The figure shows three views and two pictorial views of one solid part (mm, origin at its lowest corner). Answer the questions. A direction names the side the tool comes from. Round coordinates to 2 decimals unless told otherwise and drop trailing zeros. Order: outer loops, then holes, each group sorted by start corner. A loop starts at its lowest first (then second) coordinate and runs counter-clockwise, first axis right, second up. Notation, with made-up numbers: (-10, 44) - (2, 44) arc R6 ccw to (2, 49) - close; hole circle Ø9 at (86.25, 89). An arc over 180 degrees is marked (long way). Use CSV: the item, a comma, the result in double quotes.
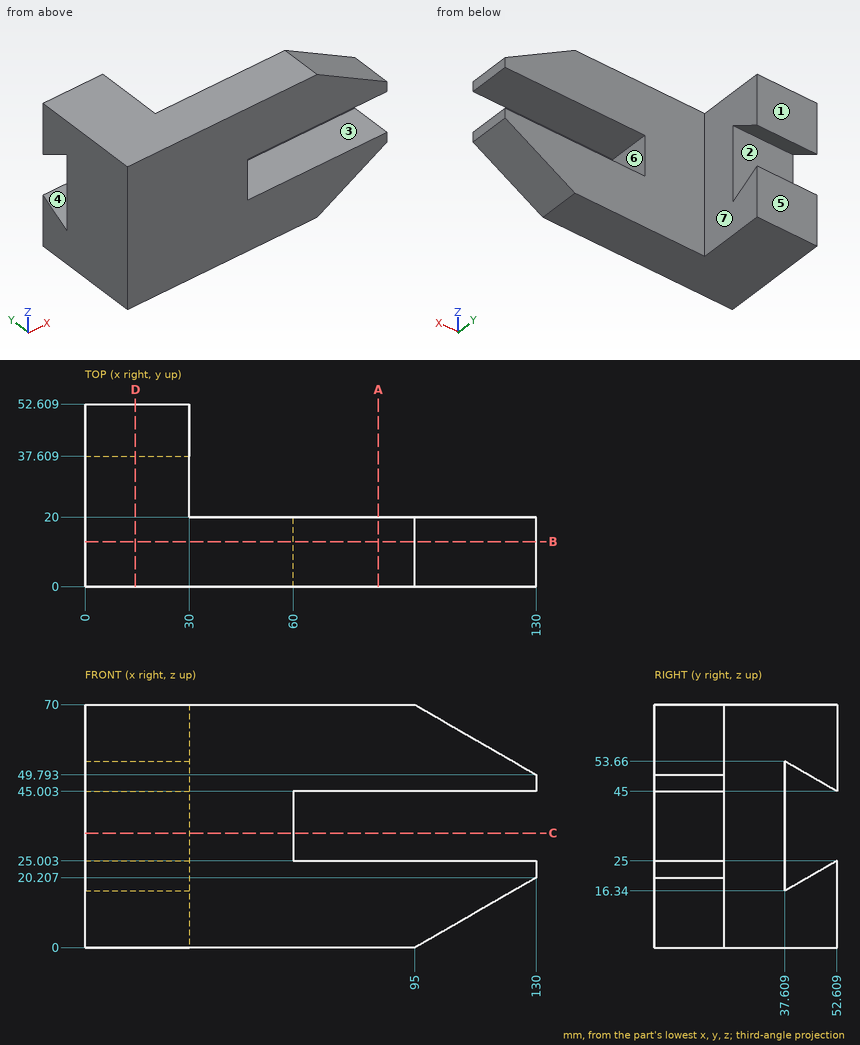
(1) Each of these flat-tipped pins is pushed along its axis until it touches: pin 1 (16 mm diameter, centred on y = 14, z = 34.5, fed in from +X); pin 2 (16.5 mm diameter, centred on y = 30.5, z = 26.5, fed in from +X); pin 3 (12 mm diameter, centred on x = 105, y = 8.5, fed in from -Z). Where does it stop, or does it pass through?
Findings below:
pin 1,"stops at x = 60"
pin 2,"stops at x = 30"
pin 3,"stops at z = 2.31"
(2) Find section D-D (x = 14.5). Determine the outline of the cut face in (y, z), and give its area (3 significant figures).
Findings below:
outline,"(0, 0) - (52.61, 0) - (52.61, 25) - (37.61, 16.34) - (37.61, 53.66) - (52.61, 45) - (52.61, 70) - (0, 70) - close"
area,"3,250 mm²"
(3) For the marked faces 5, 6 and 7, determine the directions among +Z, -Z, +X, -X, +Y, -Y from which every point of the face is accessible in a straight line to the end or side of a thin tool.
Findings below:
face 5,"+Z, -Z, +X, -X, +Y"
face 6,"+X, +Y, -Y"
face 7,"+Z, -Z, +X, +Y"
(4) Find section C-C (z = 33). Determine the outline of the cut face in (x, y).
Findings below:
outline,"(0, 0) - (60, 0) - (60, 20) - (30, 20) - (30, 37.61) - (0, 37.61) - close"
(5) The mould has two halves that part along Y. Classify the marked faces 1, 2, 3 and 4: released by +Y, released by -Y, zero draft, split by the parting line, or undercut.
Findings below:
face 1,"released by +Y"
face 2,"undercut"
face 3,"zero draft"
face 4,"undercut"
(6) Find the intervals of material crossed by L1, parallel to Z at x = 74.5, y = 15.5; L2, parallel to X at y = 48.5, z = 57.5; L3, parallel to Y at x = 72, z = 49, in increasing order. Write a range as from..to.
Findings below:
L1,"z = 0..25, 45..70"
L2,"x = 0..30"
L3,"y = 0..20"
(7) Find section A-A (x = 84.5). Determine the outline of the cut face in (y, z), and give its area (3 significant figures).
Findings below:
outline,"(0, 0) - (20, 0) - (20, 25) - (0, 25) - close; (0, 45) - (20, 45) - (20, 70) - (0, 70) - close"
area,"1,000 mm²"
(8) Find section B-B (y = 13). Determine the outline of the cut face in (x, z), and give its area (3 significant figures).
Findings below:
outline,"(0, 0) - (95, 0) - (130, 20.21) - (130, 25) - (60, 25) - (60, 45) - (130, 45) - (130, 49.79) - (95, 70) - (0, 70) - close"
area,"6,990 mm²"
